Design review of the part built by this model. Coordinates are the model's own, in mm. A direction names the side the tool comes from. Coordinates: 2 decimals unless noted, no trailing zeros. Write each loop counter-clockwise with the first axis right and the second up, starting at its lowest first coordinate (ties: lowest second). Pieces come first, ordered by that corner, then holes.
Q1. For probe 1 along Y at (x, z) = (28.25, 18); probe 2 along Y at (x, z) = (21, 1.8); probe 3 along Y at (x, z) = (6, 2.1), list the stretches that pass through material, from the lowest coordinate up.
Q2. Machinability: for faces 1 (the flat face through (5, 22, 2)), 2 (the flat face through (29, 38, 33)), 3 (the flat face through (28, 22, 28)), 4 (the flat face through (0, 38, 1)), 5 (the flat face through (27, 25, 19)), which of the approach directions +Z, -Z, +X, -X, +Y, -Y give a long, thin tool a straight path to every point of the face, cutting with its end or side? Answer none if there is none.
Q3. Take a section at D-D (x = 6). Give the boundary of the cut face in (y, z).
Q4. Take a section at B-B (x = 21). Give the boundary of the cut face in (y, z), and give its area (3 significant figures).
Q5. Take a section at A-A (z = 18). Give the boundary of the cut face in (x, y).
Q6. Take a section at C-C (y = 10). Give the boundary of the cut face in (x, z).
Q7. Mouldability with a two-part tool opening along X and no side actions: class faces 6 (the cylindrical face through (20.733, 41.033, 1.479)), 7 (the flat face through (10.2, 24, 2)), 8 (the cylindrical face through (19.373, 8.753, 1.479)), 9 (the flat face through (27.3, 0, 9.1)) as pulls with the +X half, pulls with the -X half, needs draft (parallel to the pull), parting line crosses it, or undercut.
Q8. Insertion check: pin 1 (5 mm diameter, centred on y = 21, z = 21.5, fed in from -X); pin 2 (0.9 mm diameter, centred on x = 28, y = 25.5, fed in from +Z); pin 3 (0.9 mm diameter, centred on y = 25.5, z = 1.5, fed in from -X); pin 4 (1 mm diameter, centred on x = 26, z = 13, fed in from -Y). Each pin has a flat end and moves straight along its axis. Give the tip position at first contact, or say it passes through.
```python
from build123d import *

# Parameters (mm, degrees)
SKETCH2_W               = 27
SKETCH2_H               = 49
SKETCH2_R               = 2.05
BOSS_EXTRUDE1_DEPTH     = 3
BOSS_EXTRUDE2_DEPTH     = 49
SKETCH5_R               = 6
CUT_EXTRUDE1_DEPTH      = 4
FILLET1_R               = 1
SKETCH6_W               = 13.2
SKETCH6_H               = 5
CUT_EXTRUDE2_DEPTH      = 4
SKETCH7_W               = 10.2
SKETCH7_H               = 5
CUT_EXTRUDE3_DEPTH      = 28
CUT_EXTRUDE3_DEPTH_BACK = 4


with BuildPart() as part:
    # Sketch2 → Boss-Extrude1 (new body)
    with BuildSketch(Plane.XY):
        with Locations((13.5, 24.5)):
            Rectangle(SKETCH2_W, SKETCH2_H)
        with Locations((6, 39)):
            Circle(SKETCH2_R, mode=Mode.SUBTRACT)
        with Locations((21, 39)):
            Circle(SKETCH2_R, mode=Mode.SUBTRACT)
        with Locations((6, 10)):
            Circle(SKETCH2_R, mode=Mode.SUBTRACT)
        with Locations((21, 10)):
            Circle(SKETCH2_R, mode=Mode.SUBTRACT)
    extrude(amount=BOSS_EXTRUDE1_DEPTH)

    # Sketch4 → Boss-Extrude2 (add)
    with BuildSketch(Plane(origin=(0, 49, 0), x_dir=(1, 0, 0), z_dir=(0, 1, 0))):
        with BuildLine():
            Line((30, -3), (30, -33))
            Line((30, -33), (27, -33))
            Line((27, -33), (27, 0))
            ThreePointArc((27, 0), (29.121320344, -0.878679656), (30, -3))
        make_face()
    extrude(amount=-BOSS_EXTRUDE2_DEPTH)

    # Sketch5 → Cut-Extrude1 (cut, through all)
    with BuildSketch(Plane.ZY.offset(-27)):
        with Locations((18, 39)):
            Circle(SKETCH5_R)
        with Locations((18, 10)):
            Circle(SKETCH5_R)
    extrude(amount=-CUT_EXTRUDE1_DEPTH, mode=Mode.SUBTRACT)

    # Fillet1
    fillet1_edges = [part.edges().sort_by_distance(p)[0] for p in [
        (27, 24.5, 3),
    ]]
    fillet(fillet1_edges, radius=FILLET1_R)

    # Sketch6 → Cut-Extrude2 (cut, through all)
    with BuildSketch(Plane.XY.offset(3)):
        with Locations((3.6, 24.5)):
            Rectangle(SKETCH6_W, SKETCH6_H)
    extrude(amount=-CUT_EXTRUDE2_DEPTH, mode=Mode.SUBTRACT)

    # Sketch7 → Cut-Extrude3 (cut, two sides)
    with BuildSketch(Plane.ZY.offset(-27)) as cut_extrude3_sk:
        with Locations((27.9, 24.5)):
            Rectangle(SKETCH7_W, SKETCH7_H)
    extrude(amount=CUT_EXTRUDE3_DEPTH, mode=Mode.SUBTRACT)
    extrude(cut_extrude3_sk.sketch, amount=-CUT_EXTRUDE3_DEPTH_BACK, mode=Mode.SUBTRACT)


solid = part.part
```
Response:
1. probe 1: y = 0 to 4, 16 to 33, 45 to 49
1. probe 2: y = 0 to 7.95, 12.05 to 36.95, 41.05 to 49
1. probe 3: y = 0 to 7.95, 12.05 to 22, 27 to 36.95, 41.05 to 49
2. face 1: +Z, -Z, -X
2. face 2: +Z, +X, -X, +Y, -Y
2. face 3: +Z, +X, -X
2. face 4: +Z, -Z, -X, +Y, -Y
2. face 5: +Z, -X, +Y, -Y
3. outline: (0, 0) - (7.95, 0) - (7.95, 3) - (0, 3) - close; (12.05, 0) - (22, 0) - (22, 3) - (12.05, 3) - close; (27, 0) - (36.95, 0) - (36.95, 3) - (27, 3) - close; (41.05, 0) - (49, 0) - (49, 3) - (41.05, 3) - close
4. outline: (0, 0) - (7.95, 0) - (7.95, 3) - (0, 3) - close; (12.05, 0) - (36.95, 0) - (36.95, 3) - (12.05, 3) - close; (41.05, 0) - (49, 0) - (49, 3) - (41.05, 3) - close
4. area: 122 mm2
5. outline: (27, 0) - (30, 0) - (30, 4) - (27, 4) - close; (27, 16) - (30, 16) - (30, 33) - (27, 33) - close; (27, 45) - (30, 45) - (30, 49) - (27, 49) - close
6. outline: (0, 0) - (3.95, 0) - (3.95, 3) - (0, 3) - close; (8.05, 0) - (18.95, 0) - (18.95, 3) - (8.05, 3) - close; (23.05, 0) - (27, 0) arc R3 ccw to (30, 3) - (30, 12) - (27, 12) - (27, 4) arc R1 cw to (26, 3) - (23.05, 3) - close; (27, 24) - (30, 24) - (30, 33) - (27, 33) - close
7. face 6: undercut
7. face 7: pulls with the -X half
7. face 8: undercut
7. face 9: needs draft
8. pin 1: stops at x = 27
8. pin 2: stops at z = 22.8
8. pin 3: stops at x = 10.2
8. pin 4: passes through
